Here's how the part is built. I have some questions about the finished solid (model axes, mm). A direction names the side the tool comes from. Give positions to 0.01 mm unless a question says otherwise; leave off trailing zeros. Order: outer loops, then holes, each group sorted by start corner. A loop starts at its lowest first (then second) coordinate and runs counter-clockwise, first axis right, second up. Notation, with made-up numbers: (-10.5, 78.25) -> (27.5, 78.25) arc R31 cw to (27.5, 117.25) -> close; hole circle Ø11 at (2.25, 32). An arc over 180 degrees is marked (long way). Write each question's results on one line, items separated by ' | '. Start each with the question number.
Q1. Imagine slicing it at A-A, the plane y = 0.25. Please give me the cut outline in (x, z), then the cut area to 3 significant figures.
Q2. Thinking about a two-plate mould opening in Z: for faces 4 (the face through (-9, 1.25, 1)), 5 (the face through (-8.434, 3.785, 1.37)), 6 (the face through (0, -1, 3)), 7 (the face through (-6.35, 3, 2)), which applies, pulls with the +Z half, pulls with the -Z half, needs draft (parallel to the pull), parting line crosses it, or undercut?
Q3. I'm going to push a flat-ended pin straight in: pin 1 (0.6 mm diameter, centred on x = 9.5, z = 1.5, fed in from +Y). Where does the tip first touch, or does it pass through?
Q4. Imagine slicing it at B-B, the plane y = 3.5. Please give me the cut outline in (x, z) (3 decimals), then the cut area to 3 significant figures.
Q5. I need wall thicknesses on line 1 along X through (y, z) = (2.55, 1.5) (3 decimals); line 2 along X through (y, z) = (2.75, 2.6); line 3 along X through (y, z) = (3.5, 2.15). Which ranges of each line are inside material? Lowest first, please. Write a range as [from, to].
Q6. For faces 1 (the face through (0, -0.1, 2)), 2 (the face through (9, 1.25, 1)), 3 (the face through (8.7, 6.25, 0.5)), which set-ups out of +Z, -Z, +X, -X, +Y, -Y let a thin tool reach every point of the face, with its end or its side?
Q7. Imagine slicing it at C-C, the plane z = 0.25. Please give me the cut outline in (x, y), then the cut area to 3 significant figures.
Q8. Imagine slicing it at D-D, the plane x = -1.75. Please give me the cut outline in (y, z).
```python
from build123d import *

# Parameters (mm, degrees)
SKETCH1_W           = 25
SKETCH1_H           = 12.5
BOSS_EXTRUDE1_DEPTH = 3
SKETCH2_W           = 12.7
SKETCH2_H           = 6.35
CUT_EXTRUDE1_DEPTH  = 3
SKETCH3_R           = 1
CUT_EXTRUDE2_DEPTH  = 5
SKETCH4_R           = 1
CUT_EXTRUDE3_DEPTH  = 5


with BuildPart() as part:
    # Sketch1 → Boss-Extrude1 (new body)
    with BuildSketch(Plane.XY):
        Rectangle(SKETCH1_W, SKETCH1_H)
    extrude(amount=BOSS_EXTRUDE1_DEPTH)

    # Sketch2 → Cut-Extrude1 (cut)
    with BuildSketch(Plane.XY.offset(3)):
        with Locations((0, 3.075)):
            Rectangle(SKETCH2_W, SKETCH2_H)
    extrude(amount=-CUT_EXTRUDE1_DEPTH, mode=Mode.SUBTRACT)

    # Sketch3 → Cut-Extrude2 (cut)
    with BuildSketch(Plane(origin=(0, 6.25, 0), x_dir=(1, 0, 0), z_dir=(0, 1, 0))):
        with Locations(Location((-9.425, -1.5, 0), (0, 0, 270))):
            Circle(SKETCH3_R)
    extrude(amount=-CUT_EXTRUDE2_DEPTH, mode=Mode.SUBTRACT)

    # Sketch4 → Cut-Extrude3 (cut)
    with BuildSketch(Plane(origin=(0, 6.25, 0), x_dir=(1, 0, 0), z_dir=(0, 1, 0))):
        with Locations(Location((9.425, -1.5, 0), (0, 0, 270))):
            Circle(SKETCH4_R)
    extrude(amount=-CUT_EXTRUDE3_DEPTH, mode=Mode.SUBTRACT)


solid = part.part
```
Geometry check:
1) outline: (-12.5, 0) -> (-6.35, 0) -> (-6.35, 3) -> (-12.5, 3) -> close; (6.35, 0) -> (12.5, 0) -> (12.5, 3) -> (6.35, 3) -> close | area: 36.9 mm²
2) face 4: undercut | face 5: undercut | face 6: pulls with the +Z half | face 7: needs draft
3) pin 1: y = 1.25
4) outline: (-12.5, 0) -> (-6.35, 0) -> (-6.35, 3) -> (-12.5, 3) -> close; (6.35, 0) -> (12.5, 0) -> (12.5, 3) -> (6.35, 3) -> close; hole circle Ø2 at (-9.425, 1.5); hole circle Ø2 at (9.425, 1.5) | area: 30.6 mm²
5) line 1: [-12.5, -10.425], [-8.425, -6.35], [6.35, 8.425], [10.425, 12.5] | line 2: [-12.5, -6.35], [6.35, 12.5] | line 3: [-12.5, -10.18], [-8.67, -6.35], [6.35, 8.67], [10.18, 12.5]
6) face 1: +Z, -Z, +Y | face 2: +Y | face 3: +Z, -Z, +X, -X, +Y
7) outline: (-12.5, -6.25) -> (12.5, -6.25) -> (12.5, 6.25) -> (6.35, 6.25) -> (6.35, -0.1) -> (-6.35, -0.1) -> (-6.35, 6.25) -> (-12.5, 6.25) -> close | area: 232 mm²
8) outline: (-6.25, 0) -> (-0.1, 0) -> (-0.1, 3) -> (-6.25, 3) -> close
